Verification items for the finished model (mm, model axes). A direction names the side the tool comes from. Round coordinates to 2 decimals unless told otherwise and drop trailing zeros. Write each loop counter-clockwise with the first axis right and the second up, starting at its lowest first coordinate (ties: lowest second). Pieces come first, ordered by that corner, then holes. Notation, with made-up numbers: (22.25, 46.25) - (40.25, 46.25) arc R32 ccw to (40.25, 83.25) - close; hole circle Ø1 at (72.25, 28). An arc over 180 degrees is marked (long way). Write each question's results on one line, items separated by ' | '.
```python
from build123d import *

# Parameters (mm, degrees)
BOSS_EXTRU_5_START       = 146
BOSS_EXTRU_5_DEPTH       = 71.6
ENL_V_START              = 143
ENL_V_MAT_EXTRU_16_DEPTH = 68.8
ENL_V_MAT_EXTRU_17_DEPTH = 12.75


with BuildPart() as part:
    # Esquisse21 → Boss.-Extru.5 (new body)
    with BuildSketch(Plane.XY.offset(BOSS_EXTRU_5_START)):
        Polygon((0, 61.14881388), (36.516512378, 61.14881388), (7.78303179, 3.954740649), (0, 3.954740649), (-7.78303179, 3.954740649), (-36.516512378, 61.14881388), align=None)
    extrude(amount=-BOSS_EXTRU_5_DEPTH)

    # Esquisse25 → Enlèv. mat.-Extru.16 (cut)
    with BuildSketch(Plane.XY.offset(ENL_V_START)):
        Polygon((-19.487098976, 47.02133199), (20.512901024, 47.02133199), (20.512901024, 49.136323087), (29.516512378, 61.14881388), (-29.516512378, 61.14881388), (-19.487098976, 49.136323087), align=None)
    extrude(amount=-ENL_V_MAT_EXTRU_16_DEPTH, mode=Mode.SUBTRACT)

    # Esquisse28 → Enlèvement de matière-Révolution1 (revolve, cut)
    with BuildSketch(Plane.XY):
        Polygon((0, 80), (0, -62.094926462), (151.911852074, -62.094926462), (151.911852074, 8.180052285), (60, 80), align=None)
    revolve(axis=Axis((0, 178.385130013, 0), (0, -1, 0)), mode=Mode.SUBTRACT)

    # Esquisse29 → Enlèv. mat.-Extru.17 (cut, symmetric)
    with BuildSketch(Plane(origin=(0, 0, 0), x_dir=(0, 0, -1), z_dir=(1, 0, 0))):
        Polygon((-140.809307475, 42.678321443), (-140.809307475, 21.477456774), (-113.038923412, 42.678321443), align=None)
    extrude(amount=ENL_V_MAT_EXTRU_17_DEPTH, both=True, mode=Mode.SUBTRACT)


solid = part.part
```
(1) Set-up check for faces 4 (the flat face through (0, 32, 140.809)), 5 (the flat face through (1, 43, 146)), 6 (the flat face through (-19.487, 48, 121)): record each of +Z, -Z, +X, -X, +Y, -Y from which the full face is reachable in a straight line by a thin tool's end or side.
Answer:
face 4: none | face 5: +Z, +X, -X, +Y, -Y | face 6: -Z, +Y
(2) Mould release check, pull along Z, two halves, no side actions. Record for faces 1 (the flat face through (-12.75, 35, 130)), 2 (the flat face through (0, 54, 143)), 3 (the flat face through (-29.544, 47.27, 126.988)): released by +Z, released by -Z, zero draft, split by the parting line, or undercut.
Answer:
face 1: undercut | face 2: released by -Z | face 3: zero draft
(3) Section check B-B (y = 48). Record the cut outline in (x, z), plus the area to 3 significant figures.
Answer:
outline: (-29.91, 96.42) arc R100.95 cw to (-19.49, 99.05) - (-19.49, 143) - (20.51, 143) - (20.51, 98.85) arc R100.95 cw to (29.91, 96.42) - (29.91, 146) - (-29.91, 146) - close | area: 1,080 mm2
(4) Thickness scan on L1, parallel to Y at x = -9.5, z = 132; L2, parallel to Z at x = -18.5, y = 56; L3, parallel to Y at x = 20, z = 123. Record the ranges inside material, lowest first.
Answer:
L1: 23.47 to 28.2, 42.68 to 47.02 | L2: 143 to 146 | L3: 29.51 to 47.02
(5) Section check A-A (y = 40.5). Record the cut outline in (x, z), plus the area to 3 significant figures.
Answer:
outline: (-26.14, 107.41) arc R110.55 cw to (26.14, 107.41) - (26.14, 146) - (-26.14, 146) - close; hole (-12.75, 115.89) - (12.75, 115.89) - (12.75, 140.81) - (-12.75, 140.81) - close | area: 1,270 mm2
(6) Go/stop test with flat-tipped pins: pin 1 Ø2.5 at (y, z) = (47.5, 116) entering from -X; pin 2 Ø5 at (x, z) = (21.5, 102) entering from +Y; pin 3 Ø17 at (y, z) = (30, 127.5) entering from -X; pin 4 Ø12 at (x, y) = (-29, 45.5) entering from +Z. Record where each tip stops, or that it passes through.
Answer:
pin 1: x = -30.29 | pin 2: y = 53.79 | pin 3: x = -25.14 | pin 4: z = 146
